Here's how the part is built. I have some questions about the finished solid (model axes, mm). Face numbers are marked on the shaded views. A direction names the side the tool comes from. Coordinates: 2 decimals unless noted, no trailing zeros. Write each loop counter-clockwise with the first axis right and the second up, starting at its lowest first coordinate (ties: lowest second). Pieces come first, ordered by that corner, then holes. Notation, with made-up numbers: M 64.25,87 L 110.25,87 A17 ccw 110.25,98 Z; hole C -19,48.25 d4. An arc over 180 degrees is marked long. Use one line per item in the form item = value. Start each with the question number.
1. Please list where these lines run through material, in increasing order: line 1 along Y through (x, z) = (9, 2.25); line 2 along X through (y, z) = (-9.5, 7.5); line 3 along Z through (x, y) = (-14, -12.75). Write a range as [from, to].
2. I want a section at B-B, the plane z = 17. List the corners of the cut face in (x, y) for me.
3. I'm going to push flat-ended pins straight in: pin 1 Ø2 at (x, z) = (7.5, 16.5) entering from -Y; pin 2 Ø2 at (x, y) = (6, 10.5) entering from -Z; pin 3 Ø5.5 at (y, z) = (-6.5, 47) entering from +X. Where does each tip first touch, or does it pass through?
4. On a 3-axis mill with a long thin cutter (end or side, diameter ignored), from which of +Z, -Z, +X, -X, +Y, -Y can I reach the whole of each face in a straight line? I mean the marked faces 1, 2, 3, 4 and 5. Say none if no direction works.
5. I want a section at A-A, the plane z = 8. List the corners of the cut face in (x, y) for me.
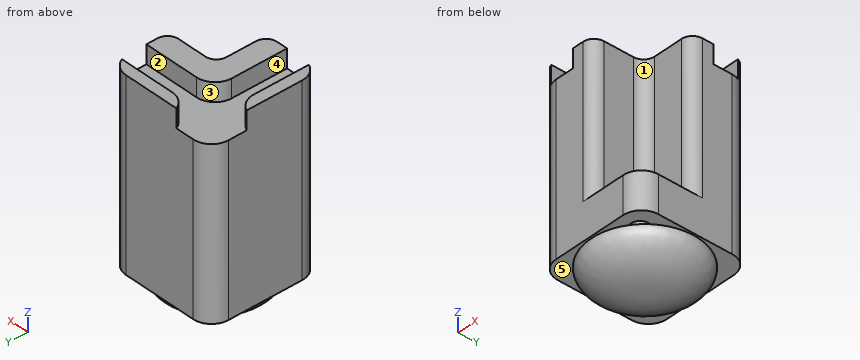
from build123d import *

# Parameters (mm, degrees)
F0_W         = 30
F0_H         = 30
F1_DEPTH     = 10
F3_DEPTH     = 40
F4_W         = 7
F4_H         = 3
F4_W_2       = 3
F4_H_2       = 7
F4_H_3       = 20
F4_W_3       = 20
F5_DEPTH     = 5
F6_R         = 2.5
F7_DEPTH     = 10
F10_R        = 5
F11_T1_DEPTH = 17.5
F11_T3_DEPTH = 16.4564392374
F12_R        = 3


# Not quite as in the source:
# - a fillet or chamfer that OpenCascade refuses, or shapes differently, is made with other operations: its cross-section is extruded or revolved along the edge and cut away or added


with BuildPart() as f1:
    # F0 (on Top) → F1 (new body)
    with BuildSketch(Plane.XY):
        Rectangle(F0_W, F0_H)
    extrude(amount=F1_DEPTH)

    # F2 (on face) → F3 (join)
    with BuildSketch(Plane.XY.offset(10)):
        Polygon((15, 15), (-15, 15), (-15, -15), (1, -15), (1, -1), (15, -1), align=None)
    extrude(amount=F3_DEPTH)

    # F4 (on face) → F5 (cut)
    with BuildSketch(Plane.XY.offset(50)):
        with Locations((-8.5, 13.5)):
            Rectangle(F4_W, F4_H)
        with Locations((-13.5, 13.5)):
            Rectangle(F4_W_2, F4_H)
        with Locations((-8.5, 8.5)):
            Rectangle(F4_W, F4_H_2)
        with Locations((-13.5, 8.5)):
            Rectangle(F4_W_2, F4_H_2)
        with Locations((-8.5, -5)):
            Rectangle(F4_W, F4_H_3)
        with Locations((5, 8.5)):
            Rectangle(F4_W_3, F4_H_2)
    extrude(amount=-F5_DEPTH, mode=Mode.SUBTRACT)

    # F6 (on face) → F7 (cut, through all)
    with BuildSketch(Plane.XY.offset(10)):
        with Locations((9, -9.5)):
            Circle(F6_R)
    extrude(amount=-F7_DEPTH, mode=Mode.SUBTRACT)

    # F8 (on Front) → F9 (revolve)
    with BuildSketch(Plane.XZ):
        with BuildLine():
            Line((0, 0), (-14.5, 0))
            add(Edge.make_bspline(
                [(-14.5, 0), (-14.5131281167, -2.1023036255), (-8.5269566385, -5.7796890584), (-3.0055961106, -6.062279921), (0, -6.0380934738)],
                knots=[0, 0, 0, 0, 0.4748413397, 1, 1, 1, 1], degree=3))
            Line((0, -6.0380934738), (0, 0))
        make_face()
    revolve(axis=Axis((0, 0, -7.25), (0, 0, -1)))

    # F10
    f10_edges = [f1.edges().sort_by_distance(p)[0] for p in [
        (-15, -15, 25),
        (15, -15, 5),
        (-15, 15, 22.5),
        (15, 15, 25),
    ]]
    fillet(f10_edges, radius=F10_R)

    # F11: fillet of radius 5 on 3 edges, made by hand

    # F11_s2 → F11_t1 (cut)
    with BuildSketch(Plane.XY.offset(45)):
        with BuildLine():
            ThreePointArc((-5, 0), (-3.5355339059, 3.5355339059), (0, 5))
            Line((0, 5), (-5, 5))
            Line((-5, 5), (-5, 0))
        make_face()
    extrude(amount=F11_T1_DEPTH, mode=Mode.SUBTRACT)

    # F11_s4 → F11_t3 (cut)
    with BuildSketch(Plane.XY.offset(45)):
        with BuildLine():
            ThreePointArc((-5, 15), (-3.1560370926, 12.8166998673), (-0.417424305, 12))
            Line((-0.417424305, 12), (-5, 12))
            Line((-5, 12), (-5, 15))
        make_face()
        with BuildLine():
            ThreePointArc((-12, 0.417424305), (-12.8166998673, 3.1560370926), (-15, 5))
            Line((-15, 5), (-12, 5))
            Line((-12, 5), (-12, 0.417424305))
        make_face()
    extrude(amount=F11_T3_DEPTH, mode=Mode.SUBTRACT)

    # F12
    f12_edges = [f1.edges().sort_by_distance(p)[0] for p in [
        (1, -1, 30),
        (1, -15, 30),
        (15, -1, 30),
    ]]
    fillet(f12_edges, radius=F12_R)


solid = f1.part
Answer list:
q1.line_1 = [-15, -12], [-7, 15]
q1.line_2 = [-15, 6.5], [11.5, 15]
q1.line_3 = [0, 50]
q2.outline = M -15,-10 A5 ccw -10,-15 L -2,-15 A3 ccw 1,-12 L 1,-4 A3 cw 4,-1 L 12,-1 A3 ccw 15,2 L 15,10 A5 ccw 10,15 L -10,15 A5 ccw -15,10 Z
q3.pin_1 = -1
q3.pin_2 = -3.89
q3.pin_3 = 1.01
q4.face_1 = +Z, +X, -Y
q4.face_2 = +Z, +X, -X
q4.face_3 = +Z
q4.face_4 = +Z, +Y, -Y
q4.face_5 = -Z
q5.outline = M -15,-10 A5 ccw -10,-15 L 10,-15 A5 ccw 15,-10 L 15,10 A5 ccw 10,15 L -10,15 A5 ccw -15,10 Z; hole C 9,-9.5 d5
